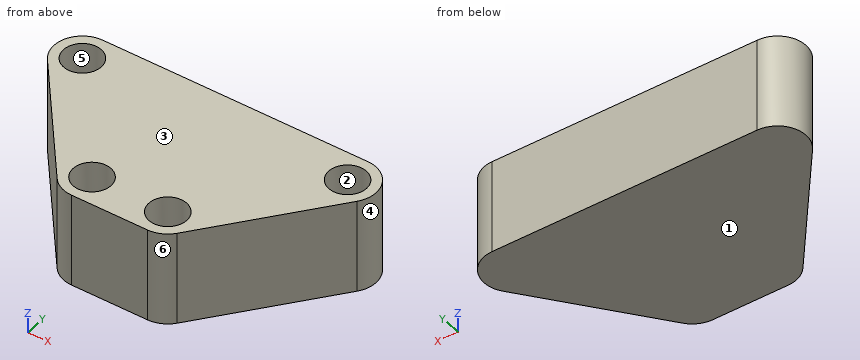
from build123d import *

# Parameters (mm, degrees)
EXTRUDE_1_DEPTH     = 25
SKETCH_2_R          = 5
CUT_EXTRUDE_1_DEPTH = 10


with BuildPart() as part:
    # 草图1 → 凸台-拉伸1 (new body)
    with BuildSketch(Plane.XY):
        with BuildLine():
            Line((0, -7.5), (20, -7.5))
            ThreePointArc((20, -7.5), (23.247595264, -6.760408641), (25.854685623, -4.6875))
            Line((25.854685623, -4.6875), (50.854685623, 26.537489992))
            ThreePointArc((50.854685623, 26.537489992), (51.760408641, 34.472585256), (45, 38.724989992))
            Line((45, 38.724989992), (-25, 38.724989992))
            ThreePointArc((-25, 38.724989992), (-31.760408641, 34.472585256), (-30.854685623, 26.537489992))
            Line((-30.854685623, 26.537489992), (-5.854685623, -4.6875))
            ThreePointArc((-5.854685623, -4.6875), (-3.247595264, -6.760408641), (0, -7.5))
        make_face()
    extrude(amount=EXTRUDE_1_DEPTH)

    # 草图2 → 切除-拉伸1 (cut)
    with BuildSketch(Plane.XY.offset(25)):
        with Locations((-25, 31.224989992)):
            Circle(SKETCH_2_R)
        Circle(SKETCH_2_R)
        with Locations((20, 0)):
            Circle(SKETCH_2_R)
        with Locations((45, 31.224989992)):
            Circle(SKETCH_2_R)
    extrude(amount=-CUT_EXTRUDE_1_DEPTH, mode=Mode.SUBTRACT)


solid = part.part
Could you check a few things on this model? Use its own coordinates, in mm. Face numbers are marked on the shaded views. A direction names the side the tool comes from. Round coordinates to 2 decimals unless told otherwise and drop trailing zeros. Order: outer loops, then holes, each group sorted by start corner. A loop starts at its lowest first (then second) coordinate and runs counter-clockwise, first axis right, second up. Notation, with made-up numbers: M 19,45 L 57,45 A22 cw 57,70 Z; hole C 69.5,-6.75 d2. An arc over 180 degrees is marked long. One line per item, written item: value.
(1) I need wall thicknesses on line 1 along X through (y, z) = (31, 16.75); line 2 along Y through (x, z) = (-24, 16); line 3 along Y through (x, z) = (45, 21.25). Which ranges of each line are inside material? Lowest first, please. Write a range as from..to.
Ans:
line 1: x = -32.5..-29.99, -20.01..40.01, 49.99..52.5
line 2: y = 17.98..26.33, 36.12..38.72
line 3: y = 19.22..26.22, 36.22..38.72
(2) Which directions (+Z, -Z, +X, -X, +Y, -Y) give clear straight access to the entire face, cutting with the end or side of a thin tool? Please do the marked faces 1 and 2.
Ans:
face 1: -Z, +X, -X, +Y, -Y
face 2: +Z
(3) Imagine slicing it at B-B (z = 23.5). Write out the boundary of the cut face in (x, y), and give its area (3 significant figures).
Ans:
outline: M -30.85,26.54 L -5.85,-4.69 A7.5 ccw 0,-7.5 L 20,-7.5 A7.5 ccw 25.85,-4.69 L 50.85,26.54 A7.5 ccw 45,38.72 L -25,38.72 A7.5 ccw Z; hole C -25,31.22 d10; hole C 0,0 d10; hole C 20,0 d10; hole C 45,31.22 d10
area: 2,540 mm^2
(4) Imagine slicing it at C-C (y = 3). Write out the boundary of the cut face in (x, z).
Ans:
outline: M -12.01,0 L 32.01,0 L 32.01,25 L 24,25 L 24,15 L 16,15 L 16,25 L 4,25 L 4,15 L -4,15 L -4,25 L -12.01,25 Z
(5) Imagine slicing it at A-A (z = 11). Write out the boundary of the cut face in (x, y), and give its area (3 significant figures).
Ans:
outline: M -30.85,26.54 L -5.85,-4.69 A7.5 ccw 0,-7.5 L 20,-7.5 A7.5 ccw 25.85,-4.69 L 50.85,26.54 A7.5 ccw 45,38.72 L -25,38.72 A7.5 ccw Z
area: 2,860 mm^2
(6) I'm going to push flat-ended pins straight in: P1, Ø10, axis at x = -22.5, z = 7, coming from the -Y side; P2, Ø1.5, axis at y = 5.5, z = 14, coming from the -X side; P3, Ø4, axis at y = 2, z = 8.5, coming from the -X side. Where does each tip first touch, or does it pass through?
Ans:
P1: stops at y = 9.86
P2: stops at x = -14.61
P3: stops at x = -12.81
(7) If we mould it in two halves opening along Y, with no side actions, what happens to the marked faces 3, 4, 5 and 6? For each: released by +Y, released by -Y, zero draft, split by the parting line, or undercut.
Ans:
face 3: zero draft
face 4: split by the parting line
face 5: undercut
face 6: released by -Y
(8) Imagine slicing it at D-D (x = 34). Write out the boundary of the cut face in (y, z).
Ans:
outline: M 5.49,0 L 38.72,0 L 38.72,25 L 5.49,25 Z
